Design review of the part built by this model. Coordinates are the model's own, in mm. A direction names the side the tool comes from. Round coordinates to 2 decimals unless told otherwise and drop trailing zeros. Loops run counter-clockwise (first coordinate to the right, second up) from the corner with the lowest first, then second, coordinate; pieces in that order, holes last. Notation, with made-up numbers: M 71.5,45.5 L 111.5,45.5 A31 ccw 111.5,70.5 Z; hole C 26,71 d7. An arc over 180 degrees is marked long. Use a Markdown table: item, result.
from build123d import *

# Parameters (mm, degrees)
BOSS_EXTRUDE1_DEPTH = 13.97
CHAMFER1_SIZE       = 0.79375
SKETCH3_R           = 2.4892
CUT_EXTRUDE1_DEPTH  = 36.400894057
CUT_EXTRUDE2_DEPTH  = 6.2
SKETCH5_R           = 4.064
CUT_EXTRUDE3_DEPTH  = 6.35
CHAFL_N1_SIZE       = 0.79375


with BuildPart() as part:
    # Sketch2 → Boss-Extrude1 (new body)
    with BuildSketch(Plane.XY):
        with BuildLine():
            Line((3.886144662, -6.731), (7.161260289, -1.058333333))
            Line((7.161260289, -1.058333333), (10.16, -1.058333333))
            Line((10.16, -1.058333333), (20.32, -1.058333333))
            Line((20.32, -1.058333333), (20.32, -12.7))
            Line((20.32, -12.7), (0, -12.7))
            ThreePointArc((0, -12.7), (-12.7, 0), (0, 12.7))
            Line((0, 12.7), (20.32, 12.7))
            Line((20.32, 12.7), (20.32, 1.058333333))
            Line((20.32, 1.058333333), (10.16, 1.058333333))
            Line((10.16, 1.058333333), (7.161260289, 1.058333333))
            Line((7.161260289, 1.058333333), (3.886144662, 6.731))
            Line((3.886144662, 6.731), (-3.886144662, 6.731))
            Line((-3.886144662, 6.731), (-7.772289324, 0))
            Line((-7.772289324, 0), (-3.886144662, -6.731))
            Line((-3.886144662, -6.731), (3.886144662, -6.731))
        make_face()
    extrude(amount=BOSS_EXTRUDE1_DEPTH)

    # Chamfer1
    chamfer1_edges = [part.edges().sort_by_distance(p)[0] for p in [
        (5.523702475, 3.894666667, 0),
        (0, 6.731, 0),
        (-5.829216993, 3.3655, 0),
        (-5.829216993, -3.3655, 0),
        (0, -6.731, 0),
        (5.523702475, -3.894666667, 0),
        (20.32, -1.058333333, 6.985),
        (20.32, -12.7, 6.985),
        (20.32, 12.7, 6.985),
        (20.32, 1.058333333, 6.985),
        (5.523702475, -3.894666667, 13.97),
        (0, -6.731, 13.97),
        (-5.829216993, -3.3655, 13.97),
        (-5.829216993, 3.3655, 13.97),
        (0, 6.731, 13.97),
        (5.523702475, 3.894666667, 13.97),
    ]]
    chamfer(chamfer1_edges, length=CHAMFER1_SIZE)

    # Sketch3 → Cut-Extrude1 (cut, through all)
    with BuildSketch(Plane(origin=(0, 12.7, 0), x_dir=(1, 0, 0), z_dir=(0, 1, 0))):
        with Locations(Location((12.660521603, -6.985, 0), (0, 0, 180))):
            Circle(SKETCH3_R)
    extrude(amount=-CUT_EXTRUDE1_DEPTH, mode=Mode.SUBTRACT)

    # Sketch4 → Cut-Extrude2 (cut)
    with BuildSketch(Plane(origin=(0, 12.7, 0), x_dir=(1, 0, 0), z_dir=(0, 1, 0))):
        Polygon((9.910890946, -11.7475), (15.41015226, -11.7475), (18.159782917, -6.985), (15.41015226, -2.2225), (9.910890946, -2.2225), (7.161260289, -6.985), align=None)
    extrude(amount=-CUT_EXTRUDE2_DEPTH, mode=Mode.SUBTRACT)

    # Sketch5 → Cut-Extrude3 (cut)
    with BuildSketch(Plane.XZ.offset(12.7)):
        with Locations((12.660521603, 6.985)):
            Circle(SKETCH5_R)
    extrude(amount=-CUT_EXTRUDE3_DEPTH, mode=Mode.SUBTRACT)

    # Chaflán1
    chafl_n1_edges = [part.edges().sort_by_distance(p)[0] for p in [
        (15.149721603, -1.058333333, 6.985),
        (15.149721603, 1.058333333, 6.985),
        (8.596521603, -12.7, 6.985),
    ]]
    chamfer(chafl_n1_edges, length=CHAFL_N1_SIZE)


solid = part.part
1. Take a section at B-B on y = 4.25. Give the boundary of the cut face in (x, z) (3 decimals).
Check values:
| item | result |
|---|---|
| outline | M -11.968,0 L -6.235,0 L -5.319,0.794 L -5.319,13.176 L -6.235,13.97 L -11.968,13.97 Z; M 5.319,0.794 L 6.235,0 L 20.32,0 L 20.32,13.97 L 6.235,13.97 L 5.319,13.176 Z; hole C 12.661,6.985 d4.978 |
2. The part is to be moulded in two halves that separate along Z. For faces 5 (the face through (-6.15, 3.62, 13.58)), 6 (the face through (5.55, 3.85, 6.9)), 7 (the face through (8.555, 9.643, 4.57)), say which applies: pulls with the +Z half, pulls with the -Z half, needs draft (parallel to the pull), parting line crosses it, or undercut.
Check values:
| item | result |
|---|---|
| face 5 | pulls with the +Z half |
| face 6 | needs draft |
| face 7 | undercut |
3. Take a section at A-A on x = 2. Give the boundary of the cut face in (y, z), and give its area (3 significant figures).
Check values:
| item | result |
|---|---|
| outline | M -12.7,0 L -7.52,0 L -6.73,0.79 L -6.73,13.18 L -7.52,13.97 L -12.7,13.97 Z; M 6.73,0.79 L 7.52,0 L 12.7,0 L 12.7,13.97 L 7.52,13.97 L 6.73,13.18 Z |
| area | 166 mm² |
4. Take a section at C-C on y = 10. Give the boundary of the cut face in (x, z) (1 decimal), and give its area (3 significant figures).
Check values:
| item | result |
|---|---|
| outline | M -7.8,0 L 20.3,0 L 20.3,14 L -7.8,14 Z; hole M 7.2,7 L 9.9,2.2 L 15.4,2.2 L 18.2,7 L 15.4,11.7 L 9.9,11.7 Z |
| area | 315 mm² |
5. Take a section at D-D on z = 1.75. Give the boundary of the cut face in (x, y).
Check values:
| item | result |
|---|---|
| outline | M -7.77,0 L -3.89,6.73 L 3.89,6.73 L 7.16,1.06 L 19.53,1.06 L 20.32,1.85 L 20.32,11.91 L 19.53,12.7 L 0,12.7 A12.7 ccw 0,-12.7 L 19.53,-12.7 L 20.32,-11.91 L 20.32,-1.85 L 19.53,-1.06 L 7.16,-1.06 L 3.89,-6.73 L -3.89,-6.73 Z |
6. Insertion check: pin 1 (6.5 mm diameter, centred on x = 12.66, z = 6.98, fed in from -Y); pin 2 (3 mm diameter, centred on x = 14.5, z = 8, fed in from +Y); pin 3 (8 mm diameter, centred on y = -7.5, z = 3.5, fed in from -X). Each pin has a flat end and moves straight along its axis. Give the tip position at first contact, or say it passes through.
Check values:
| item | result |
|---|---|
| pin 1 | stops at y = -6.35 |
| pin 2 | stops at y = 6.5 |
| pin 3 | stops at x = -12.21 |
7. Wall thickness on line 1 along Y through (x, z) = (0, 12.5); line 2 along X through (y, z) = (-11, 6.75); line 3 along X through (y, z) = (4.75, 5.25): over which ranges is each line inside the solid? List them lowest first. Write a range as from..to.
Check values:
| item | result |
|---|---|
| line 1 | y = -12.7..-6.73, 6.73..12.7 |
| line 2 | x = -6.35..8.6, 16.72..20.32 |
| line 3 | x = -11.78..-5.03, 5.03..10.88, 14.45..20.32 |
8. Machinability: for faces 1 (the face through (10, 6.5, 7)), 2 (the face through (-6.21, -3.51, 13.58)), 3 (the face through (5.9, 4.05, 0.39)), 4 (the face through (-5.802, 3.413, 6.898)), which of the approach directions +Z, -Z, +X, -X, +Y, -Y give a long, thin tool a straight path to every point of the face, cutting with its end or side? Answer none if there is none.
Check values:
| item | result |
|---|---|
| face 1 | +Y |
| face 2 | +Z |
| face 3 | -Z |
| face 4 | +Z, -Z |
